Geometry: final body of the model. Coordinates: model frame, mm. A direction names the side the tool comes from. Coordinates: 2 decimals unless noted, no trailing zeros. Loops run counter-clockwise (first coordinate to the right, second up) from the corner with the lowest first, then second, coordinate; pieces in that order, holes last. Notation, with made-up numbers: (45.5, 5) -> (74.5, 5) arc R12 cw to (74.5, 13) -> close; hole circle Ø6 at (59, 18). An arc over 180 degrees is marked (long way). One line per item, written item: value. Start each with the question number.
Item 1: Section query B-B on z = -49. Return loops of the section in (x, y).
Item 2: Mould query, pull axis Z, two halves, no side actions, for faces 1 (the cylindrical face through (16.45, 1.25, -9.61)), 2 (the cylindrical face through (-38.061, 1.252, 66.013)), 3 (the flat face through (0, 2.54, 10)). Classes: +Z half, -Z half, draft (parallel to the pull), parting line (faces both ways), or undercut.
Item 3: Section query A-A on x = 0. Return loops of the section in (y, z), then the cut area to 3 significant figures.
Item 4: Contact query for flat-ended pins moving along their axis: pin 1 Ø1.3 at (x, y) = (35.5, 1) entering from -Z; pin 2 Ø1.5 at (y, z) = (1.5, 48.5) entering from -X. Output: stop coordinate, or through.
Item 5: Section query D-D on z = -13. Return loops of the section in (x, y).
Item 6: Ray query, probe 1 along Z at (x, y) = (21, 0.95) (3 decimals); probe 2 along Z at (x, y) = (20, 2.05) (3 decimals); probe 3 along Z at (x, y) = (50, 0.4) (3 decimals). Return the intervals inside material, ascending. Write a range as from..to.
Item 7: Section query C-C on y = 0.45. Give the number of separate pieces and of enclosed holes in the cut face, then the cut area to 3 significant figures.
Item 8: Set-up query: faces 4 (the flat face through (-26.3, 1.3, -39.2)), 5 (the flat face through (26.68, 1.25, -39.86)), 6 (the flat face through (21.18, 1.252, 43.036)), 7 (the flat face through (20.78, 1.25, -42.34)). Return all of +Z, -Z, +X, -X, +Y, -Y with unobstructed straight access to the full face (end or side cutting, diameter ignored); none if empty.
from build123d import *

# Parameters (mm, degrees)
BOSS_EXTRUDE1_DEPTH         = 2.54
F_5_8_CLEARANCE_HOLE1_D     = 16.27124
F_5_8_CLEARANCE_HOLE1_DEPTH = 38.354
F_5_8_CLEARANCE_HOLE1_TIP   = 4.888373669
F_4_CLEARANCE_HOLE1_D       = 2.9464
F_4_CLEARANCE_HOLE1_DEPTH   = 38.354
F_4_CLEARANCE_HOLE1_TIP     = 0.885187864


with BuildPart() as part:
    # Sketch1 → Boss-Extrude1 (new body)
    with BuildSketch(Plane(origin=(0, 0, 0), x_dir=(1, 0, 0), z_dir=(0, 1, 0))):
        with BuildLine():
            Line((18.783553311, 3.175), (76.133825433, 3.175))
            ThreePointArc((76.133825433, 3.175), (76.2, 0), (76.133825433, -3.175))
            Line((76.133825433, -3.175), (18.783553311, -3.175))
            ThreePointArc((18.783553311, -3.175), (16.497783942, -9.525), (12.141407313, -14.679534341))
            Line((12.141407313, -14.679534341), (40.816543373, -64.346326912))
            ThreePointArc((40.816543373, -64.346326912), (38.1, -65.991135768), (35.317282059, -67.521326912))
            Line((35.317282059, -67.521326912), (6.642145999, -17.854534341))
            ThreePointArc((6.642145999, -17.854534341), (0, -19.05), (-6.642145999, -17.854534341))
            Line((-6.642145999, -17.854534341), (-35.317282059, -67.521326912))
            ThreePointArc((-35.317282059, -67.521326912), (-38.1, -65.991135768), (-40.816543373, -64.346326912))
            Line((-40.816543373, -64.346326912), (-12.141407313, -14.679534341))
            ThreePointArc((-12.141407313, -14.679534341), (-16.497783942, -9.525), (-18.783553311, -3.175))
            Line((-18.783553311, -3.175), (-76.133825433, -3.175))
            ThreePointArc((-76.133825433, -3.175), (-76.2, 0), (-76.133825433, 3.175))
            Line((-76.133825433, 3.175), (-18.783553311, 3.175))
            ThreePointArc((-18.783553311, 3.175), (-16.497783942, 9.525), (-12.141407313, 14.679534341))
            Line((-12.141407313, 14.679534341), (-40.816543373, 64.346326912))
            ThreePointArc((-40.816543373, 64.346326912), (-38.1, 65.991135768), (-35.317282059, 67.521326912))
            Line((-35.317282059, 67.521326912), (-6.642145999, 17.854534341))
            ThreePointArc((-6.642145999, 17.854534341), (0, 19.05), (6.642145999, 17.854534341))
            Line((6.642145999, 17.854534341), (35.317282059, 67.521326912))
            ThreePointArc((35.317282059, 67.521326912), (38.1, 65.991135768), (40.816543373, 64.346326912))
            Line((40.816543373, 64.346326912), (12.141407313, 14.679534341))
            ThreePointArc((12.141407313, 14.679534341), (16.497783942, 9.525), (18.783553311, 3.175))
        make_face()
    extrude(amount=BOSS_EXTRUDE1_DEPTH)

    # 5/8 Clearance Hole1
    with Locations(Plane(origin=(0, 2.54, 0), x_dir=(1, 0, 0), z_dir=(0, 1, 0))):
        with Locations((0, 0)):
            Hole(F_5_8_CLEARANCE_HOLE1_D / 2, depth=F_5_8_CLEARANCE_HOLE1_DEPTH)
            with Locations((0, 0, -(F_5_8_CLEARANCE_HOLE1_DEPTH + F_5_8_CLEARANCE_HOLE1_TIP / 2))):  # 118° drill point
                Cone(0, F_5_8_CLEARANCE_HOLE1_D / 2, F_5_8_CLEARANCE_HOLE1_TIP, mode=Mode.SUBTRACT)

    # #4 Clearance Hole1
    with Locations(Plane(origin=(0, 2.54, 0), x_dir=(1, 0, 0), z_dir=(0, 1, 0))):
        with Locations((-73.025, 0), (-36.5125, 63.241505111), (36.5125, 63.241505111), (73.025, 0), (36.5125, -63.241505111), (-36.5125, -63.241505111)):
            Hole(F_4_CLEARANCE_HOLE1_D / 2, depth=F_4_CLEARANCE_HOLE1_DEPTH)
            with Locations((0, 0, -(F_4_CLEARANCE_HOLE1_DEPTH + F_4_CLEARANCE_HOLE1_TIP / 2))):  # 118° drill point
                Cone(0, F_4_CLEARANCE_HOLE1_D / 2, F_4_CLEARANCE_HOLE1_TIP, mode=Mode.SUBTRACT)


solid = part.part
Reply:
1. outline: (-31.96, 0) -> (-24.62, 0) -> (-24.62, 2.54) -> (-31.96, 2.54) -> close; (24.62, 0) -> (31.96, 0) -> (31.96, 2.54) -> (24.62, 2.54) -> close
2. face 1: undercut
2. face 2: +Z half
2. face 3: draft
3. outline: (0, -19.05) -> (2.54, -19.05) -> (2.54, -8.14) -> (0, -8.14) -> close; (0, 8.14) -> (2.54, 8.14) -> (2.54, 19.05) -> (0, 19.05) -> close
3. area: 55.4 mm²
4. pin 1: stops at z = -67.52
4. pin 2: stops at x = -32.1
5. outline: (-13.92, 0) -> (13.92, 0) -> (13.92, 2.54) -> (-13.92, 2.54) -> close
6. probe 1: z = -42.723..-30.023, -3.175..3.175, 30.023..42.723
6. probe 2: z = -40.991..-28.291, -3.175..3.175, 28.291..40.991
6. probe 3: z = -3.175..3.175
7. separate pieces: 1
7. enclosed holes: 7
7. area: 3,070 mm²
8. face 4: -X, +Y, -Y
8. face 5: +X, +Y, -Y
8. face 6: +Z, +Y, -Y
8. face 7: -Z, +Y, -Y
